```python
from build123d import *

# Parameters (mm, degrees)
SKETCH11_W           = 36.88
SKETCH11_H           = 19
BOSS_EXTRUDE3_DEPTH  = 3.175
BOSS_EXTRUDE2_DEPTH  = 3.175
SKETCH4_R            = 1.025
CUT_EXTRUDE4_DEPTH   = 80.923101916
M5_CLEARANCE_HOLE1_D = 5.5
FILLET1_R            = 2.5
FILLET2_R            = 10.5


with BuildPart() as part:
    # Sketch11 → Boss-Extrude3 (new, symmetric)
    with BuildSketch(Plane(origin=(0, 0, 0), x_dir=(0, 0, -1), z_dir=(1, 0, 0))):
        with Locations((-43.587249817, -15.5)):
            Rectangle(SKETCH11_W, SKETCH11_H)
    extrude(amount=BOSS_EXTRUDE3_DEPTH, both=True)

    # Sketch8 → Boss-Extrude2 (add, symmetric)
    with BuildSketch(Plane(origin=(0, 0, 0), x_dir=(0, 0, -1), z_dir=(1, 0, 0))):
        Polygon((14.5, 10), (14.5, -50), (26.73162128, -50), (26.73162128, 22.23162128), (-26.73162128, 22.23162128), (-26.73162128, -50), (-14.5, -50), (-14.5, 10), align=None)
    extrude(amount=BOSS_EXTRUDE2_DEPTH, both=True)

    # Sketch4 → Cut-Extrude4 (cut, through all)
    with BuildSketch(Plane.ZY.offset(3.175)):
        with Locations((17.3, -39.5)):
            Circle(SKETCH4_R)
        with Locations(Location((-17.3, -39.5, 0), (0, 0, 180))):
            Circle(SKETCH4_R)
        with Locations((17.3, -17.5)):
            Circle(SKETCH4_R)
        with Locations(Location((-17.3, -17.5, 0), (0, 0, 180))):
            Circle(SKETCH4_R)
        with Locations(Location((-17.3, 4.5, 0), (0, 0, 180))):
            Circle(SKETCH4_R)
        with Locations((17.3, 4.5)):
            Circle(SKETCH4_R)
    extrude(amount=-CUT_EXTRUDE4_DEPTH, mode=Mode.SUBTRACT)

    # M5 Clearance Hole1 (through all)
    with Locations(Plane(origin=(3.175, 0, 0), x_dir=(0, 0, -1), z_dir=(1, 0, 0))):
        with Locations((-53.587249817, -15.5), (-33.587249817, -15.5)):
            Hole(M5_CLEARANCE_HOLE1_D / 2)

    # Fillet1
    fillet1_edges = [part.edges().sort_by_distance(p)[0] for p in [
        (0, -25, 26.73162128),
        (0, 22.23162128, 26.73162128),
        (0, -50, -14.5),
        (0, -50, -26.73162128),
        (0, 22.23162128, -26.73162128),
        (0, -50, 26.73162128),
        (0, -50, 14.5),
        (0, -25, 62.027249817),
        (0, -6, 62.027249817),
    ]]
    fillet(fillet1_edges, radius=FILLET1_R)

    # Fillet2
    fillet2_edges = [part.edges().sort_by_distance(p)[0] for p in [
        (0, -6, 26.73162128),
    ]]
    fillet(fillet2_edges, radius=FILLET2_R)


solid = part.part
```
Geometry check sheet. Reference: the model listing, model coordinates, mm. A direction names the side the tool comes from. Give positions to 0.01 mm unless a question says otherwise; leave off trailing zeros. Loops run counter-clockwise (first coordinate to the right, second up) from the corner with the lowest first, then second, coordinate; pieces in that order, holes last. Notation, with made-up numbers: M -38,60.5 L 9,60.5 A15 ccw 9,75.5 Z; hole C 36.5,87 d9. An arc over 180 degrees is marked long. Write item = value, one per line. Start each with the question number.
1. Section check C-C, the plane y = -26. Enter the section's corners in (x, z) (3 decimals).
2. Thickness scan on probe 1 along Y at (x, z) = (0.25, -17.3) (3 decimals); probe 2 along Z at (x, y) = (0.25, -42); probe 3 along Z at (x, y) = (1, -40). Record the ranges inside material, lowest first.
3. Section check A-A, the plane y = -15.5. Enter the section's corners in (x, z) (3 decimals).
4. Tool access check on faces 1 (the face through (0, -49, 15)), 2 (the face through (-0.04, -16.81, 16.54)), 3 (the face through (0, -6, 49)), 4 (the face through (0, -37, 26.732)), 5 (the face through (0, 21.5, -26)). Record the directions out of +Z, -Z, +X, -X, +Y, -Y that give a thin tool (end or side, any length) a straight path to the whole face; none if there is none.
5. Draft check along Y on faces 6 (the face through (3.175, -5, 18)), 7 (the face through (-0.04, -40.19, -16.54)), 8 (the face through (0, 21.5, 26)). Enter one of: +Y half, -Y half, draft (parallel to the pull), parting line (faces both ways), or undercut.
6. Go/stop test with flat-tipped pins: P1, Ø1.9, axis at x = -1, y = 11.5, coming from the +Z side; P2, Ø2, axis at x = -0.5, z = 51.5, coming from the +Y side; P3, Ø5, axis at y = -15.5, z = 53.59, coming from the +X side; P4, Ø1, axis at x = 2, y = 1.5, coming from the +Z side. Record where each tip stops, or that it passes through.
7. Section check D-D, the plane y = -39.5. Enter the section's corners in (x, z) (3 decimals), plus the area to 3 significant figures.
8. Section check B-B, the plane x = -0.75. Give the number of separate pieces and of enclosed holes in the cut face, plus the area to 3 significant figures.
Values follow:
q1.outline = M -3.175,-26.732 L 3.175,-26.732 L 3.175,-14.5 L -3.175,-14.5 Z; M -3.175,14.5 L 3.175,14.5 L 3.175,27.232 L -3.175,27.232 Z
q2.probe_1 = -50 to -40.525, -38.475 to -18.525, -16.475 to 3.475, 5.525 to 22.232
q2.probe_2 = -26.73 to -14.5, 14.5 to 26.73
q2.probe_3 = -26.73 to -18.19, -16.41 to -14.5, 14.5 to 16.41, 18.19 to 26.73
q3.outline = M -3.175,-26.732 L 3.175,-26.732 L 3.175,-14.5 L -3.175,-14.5 Z; M -3.175,14.5 L 3.175,14.5 L 3.175,30.837 L -3.175,30.837 Z; M -3.175,36.337 L 3.175,36.337 L 3.175,50.837 L -3.175,50.837 Z; M -3.175,56.337 L 3.175,56.337 L 3.175,62.027 L -3.175,62.027 Z
q4.face_1 = +X, -X, -Y
q4.face_2 = +X, -X
q4.face_3 = +Z, +X, -X, +Y
q4.face_4 = +Z, +X, -X, -Y
q4.face_5 = -Z, +X, -X, +Y
q5.face_6 = draft
q5.face_7 = undercut
q5.face_8 = +Y half
q6.P1 = 26.73
q6.P2 = -6
q6.P3 = through
q6.P4 = 27.33
q7.outline = M -3.175,-26.732 L 3.175,-26.732 L 3.175,-18.325 L -3.175,-18.325 Z; M -3.175,-16.275 L 3.175,-16.275 L 3.175,-14.5 L -3.175,-14.5 Z; M -3.175,14.5 L 3.175,14.5 L 3.175,16.275 L -3.175,16.275 Z; M -3.175,18.325 L 3.175,18.325 L 3.175,26.732 L -3.175,26.732 Z
q7.area = 129 mm^2
q8.separate_pieces = 1
q8.enclosed_holes = 8
q8.area = 2,740 mm^2
